```python
from build123d import *

# Parameters (mm, degrees)
F1_DEPTH = 30
F3_DEPTH = 20
F4_SIZE  = 5
F6_DEPTH = 100


with BuildPart() as f1:
    # F0 (on Top) → F1 (new body)
    with BuildSketch(Plane.XY):
        Polygon((-55.034131, 29.962024), (-55.034131, 0), (-55.034131, -29.884199), (15.098164, -29.884199), (40.813338, 0), (15.098164, 29.962024), align=None)
    extrude(amount=F1_DEPTH)

    # F2 (on face) → F3 (cut)
    with BuildSketch(Plane(origin=(0, 0, 0), x_dir=(1, 0, 0), z_dir=(0, 0, -1))):
        Polygon((35.202757, 0), (13.929292, 24.974938), (-50.124869, 24.974938), (-50.124869, -25.754089), (13.695518, -25.754089), align=None)
    extrude(amount=-F3_DEPTH, mode=Mode.SUBTRACT)

    # F4
    f4_edges = [f1.edges().sort_by_distance(p)[0] for p in [
        (27.955751, -14.942099, 30),
        (27.955751, 14.981012, 30),
        (-19.967983, 29.962024, 30),
        (-19.967983, -29.884199, 30),
        (-55.034131, 0.038913, 30),
    ]]
    chamfer(f4_edges, length=F4_SIZE)

    # F5 (on face) → F6 (cut)
    with BuildSketch(Plane(origin=(0, 29.962024, 0), x_dir=(-1, 0, 0), z_dir=(0, 1, 0))):
        with BuildLine():
            Line((4.414184, 0), (14.482094, 0))
            ThreePointArc((14.482094, 0), (9.448139, 5.033955), (4.414184, 0))
        make_face()
    extrude(amount=-F6_DEPTH, mode=Mode.SUBTRACT)


solid = f1.part
```
Here's how the part is built. I have some questions about the finished solid (model axes, mm). A direction names the side the tool comes from. Coordinates: 2 decimals unless noted, no trailing zeros. Loops run counter-clockwise (first coordinate to the right, second up) from the corner with the lowest first, then second, coordinate; pieces in that order, holes last. Notation, with made-up numbers: (15.5, -24.75) - (26.5, -24.75) arc R13 ccw to (26.5, 0.25) - close; hole circle Ø4 at (15.5, -7.75). An arc over 180 degrees is marked (long way). Return JSON: item names as keys, results as strings. Group by question number.
Item 1: On a 3-axis mill with a long thin cutter (end or side, diameter ignored), from which of +Z, -Z, +X, -X, +Y, -Y can I reach the whole of each face in a straight line? I mean faces 4 (the face through (-9.559, -27.395, 5.033)), 5 (the face through (24.715, -12.313, 9.86)). Say none if no direction works.
Item 2: If we section it at C-C on y = -18: Write out the boundary of the cut face in (x, z).
Item 3: If we section it at A-A on z = 6.25: Write out the boundary of the cut face in (x, y), and give its area (3 significant figures).
Item 4: I need wall thicknesses on line 1 (Y direction, x = -40, z = 4.5); line 2 (Z direction, x = -20, y = 3.5); line 3 (X direction, y = -23, z = 14.75). Which ranges of each line are inside material? Lowest first, please. Write a range as from..to.
Item 5: We'd pull the mould along Y, two halves only. Please class faces 1 (the face through (-51, 0, 0)), 2 (the face through (28.136, 14.771, 12.325)), 3 (the face through (24.299, 13.057, 9.86)): +Y half, -Y half, draft (parallel to the pull), parting line (faces both ways), or undercut.
Item 6: Will these pins go through, and if not, where does the flat tip stop? P1, Ø6, axis at y = 9.5, z = 9, coming from the +X side; P2, Ø4, axis at y = 4.5, z = 24.5, coming from the +X side; P3, Ø12, axis at y = -19, z = 4.5, coming from the +X side.
Item 7: If we section it at D-D on z = 23: Write out the boundary of the cut face in (x, y).
Item 8: If we section it at B-B on x = -30: Write out the boundary of the cut face in (y, z), and give its area (3 significant figures).
Calculated:
{
 "1": {"face 4": "-Z, +Y, -Y", "face 5": "-Z"},
 "2": {"outline": "(-55.03, 0) - (-50.12, 0) - (-50.12, 20) - (19.87, 20) - (19.87, 0) - (25.32, 0) - (25.32, 25) - (18.73, 30) - (-50.03, 30) - (-55.03, 25) - close"},
 "3": {"outline": "(-55.03, -29.88) - (15.1, -29.88) - (40.81, 0) - (15.1, 29.96) - (-55.03, 29.96) - close; hole (-50.12, -24.97) - (13.93, -24.97) - (35.2, 0) - (13.7, 25.75) - (-50.12, 25.75) - close", "area": "1,180 mm^2"},
 "4": {"line 1": "y = -29.88..-24.97, 25.75..29.96", "line 2": "z = 20..30", "line 3": "x = -55.03..-50.12, 15.61..21.02"},
 "5": {"face 1": "draft", "face 2": "+Y half", "face 3": "undercut"},
 "6": {"P1": "stops at x = 35.23", "P2": "stops at x = 38.67", "P3": "stops at x = 29.63"},
 "7": {"outline": "(-55.03, -29.88) - (15.1, -29.88) - (40.81, 0) - (15.1, 29.96) - (-55.03, 29.96) - close"},
 "8": {"outline": "(-29.88, 0) - (-24.97, 0) - (-24.97, 20) - (25.75, 20) - (25.75, 0) - (29.96, 0) - (29.96, 25) - (24.96, 30) - (-24.88, 30) - (-29.88, 25) - close", "area": "756 mm^2"}
}
